```python
from build123d import *

# Parameters (mm, degrees)
SKETCH_1_R      = 2.15
EXTRUDE_1_DEPTH = 20
FILLET_1_R      = 10
FILLET_2_R      = 50
FILLET_3_R      = 1


with BuildPart() as part:
    # ｽｹｯﾁ1 → ﾎﾞｽ - 押し出し1 (new body)
    with BuildSketch(Plane(origin=(0, 0, 0), x_dir=(1, 0, 0), z_dir=(0, 1, 0))):
        with BuildLine():
            Line((-30, -24.445436483), (-19.445436483, -24.445436483))
            ThreePointArc((-19.445436483, -24.445436483), (-18.602258519, -24.373828809), (-17.78323176, -24.161056851))
            ThreePointArc((-17.78323176, -24.161056851), (0, -30), (17.78323176, -24.161056851))
            ThreePointArc((17.78323176, -24.161056851), (24.321347518, -18.338417254), (15.909902577, -15.909902577))
            Line((15.909902577, -15.909902577), (14.849242405, -14.849242405))
            ThreePointArc((14.849242405, -14.849242405), (0, -21), (-14.849242405, -14.849242405))
            Line((-14.849242405, -14.849242405), (-15.909902577, -15.909902577))
            ThreePointArc((-15.909902577, -15.909902577), (-17.532019321, -14.82603882), (-19.445436483, -14.445436483))
            Line((-19.445436483, -14.445436483), (-30, -14.445436483))
            Line((-30, -14.445436483), (-30, -24.445436483))
        make_face()
        with Locations(Location((-19.445436483, -19.445436483, 0), (0, 0, 270))):
            Circle(SKETCH_1_R, mode=Mode.SUBTRACT)
        with Locations(Location((19.445436483, -19.445436483, 0), (0, 0, 90))):
            Circle(SKETCH_1_R, mode=Mode.SUBTRACT)
    extrude(amount=EXTRUDE_1_DEPTH)

    # ﾌｨﾚｯﾄ1
    # the kernel refuses this fillet: 10 mm, written as the material it adds along each edge
    with BuildSketch(Plane(origin=(17.78323176, 0, 24.161056851), x_dir=(-0.8339213468601729, 0, 0.5518833094512962), z_dir=(0, 1, 0))) as fillet_1_piece_1:
        with BuildLine():
            CenterArc((3.490042654, 9.987563289), FILLET_1_R, 240.094065847, 27.048110546)
            ThreePointArc((-1.495732566, 1.319112133), (-0.681431037, 0.734886554), (0, 0))
            ThreePointArc((0, 0), (1.495732566, 0.037310133), (2.991465132, 0))
        make_face()
    extrude(amount=20)
    with BuildSketch(Plane(origin=(-17.78323176, 0, 24.161056851), x_dir=(-0.9938473156865714, 0, 0.11075880598217346), z_dir=(0, 1, 0))) as fillet_1_piece_2:
        with BuildLine():
            CenterArc((3.675145817, 9.938473157), FILLET_1_R, 233.085304015, 30.555636739)
            Line((-2.331107377, 1.943166873), (-2.931732696, 1.143636244))
            ThreePointArc((-2.931732696, 1.143636244), (-1.781263353, 0.232951381), (-0.678328899, -0.734758399))
            Line((-0.678328899, -0.734758399), (0.225936244, -0.974142091))
            ThreePointArc((0.225936244, -0.974142091), (1.572716444, -0.895321193), (2.456798951, -0.993847316))
            Line((2.456798951, -0.993847316), (2.567557757, 0))
        make_face()
    extrude(amount=20)
    # the kernel refuses this fillet: 10 mm, written as the material it takes off along each edge
    with BuildSketch(Plane(origin=(-14.849242405, -10.471736153, 14.849242405), x_dir=(-0.707106781186226, 0, 0.7071067811868691), z_dir=(0, 1, 0))) as fillet_1_2_piece_1:
        with BuildLine():
            CenterArc((9.383333333, 6.15248369), FILLET_1_R, 191.447340283, 26.522629156)
            ThreePointArc((-0.417741935, 4.167811532), (-0.104696468, 2.094347231), (0, 0))
            Line((0, 0), (1.5, 0))
        make_face()
    extrude(amount=40.943472307, mode=Mode.SUBTRACT)
    with BuildSketch(Plane(origin=(14.849242405, -10.471736153, 14.849242405), x_dir=(-0.7741018071953127, 0, 0.6330611282466734), z_dir=(0, 1, 0))) as fillet_1_2_piece_2:
        with BuildLine():
            CenterArc((5.186002666, 9.950144539), FILLET_1_R, 237.753700702, 26.522629156)
            Line((-0.149596231, 1.492521681), (0, 0))
            ThreePointArc((0, 0), (2.094347231, 0.104696468), (4.188694461, 0))
        make_face()
    extrude(amount=40.943472307, mode=Mode.SUBTRACT)

    # ﾌｨﾚｯﾄ2
    fillet_2_edges = [part.edges().sort_by_distance(p)[0] for p in [
        (-15.909902577, 10, 15.909902577),
        (15.909902577, 10, 15.909902577),
    ]]
    fillet(fillet_2_edges, radius=FILLET_2_R)

    # ﾌｨﾚｯﾄ3
    fillet_3_edges = [part.edges().sort_by_distance(p)[0] for p in [
        (-30, 10, 14.445436483),
        (-30, 10, 24.445436483),
    ]]
    fillet(fillet_3_edges, radius=FILLET_3_R)


solid = part.part
```
CAD build for the part. Positions are in the model's coordinates, mm. A direction names the side the tool comes from. Round coordinates to 2 decimals unless told otherwise and drop trailing zeros. Write each loop counter-clockwise with the first axis right and the second up, starting at its lowest first coordinate (ties: lowest second). Pieces come first, ordered by that corner, then holes. Notation, with made-up numbers: (38.25, 39.25) - (96.25, 39.25) arc R10 cw to (96.25, 58.25) - close; hole circle Ø10 at (6, -7.5). An arc over 180 degrees is marked (long way). Write item = value, one per line. Start each with the question number.
Q1. Band-saw the part on D-D (x = 6). Give the cut face in (y, z).
Q2. Band-saw the part on B-B (x = -18). Give the cut face in (y, z), then the cut area to 3 significant figures.
Q3. Probe L1, parallel to Z at x = 21, y = 17; L2, parallel to X at y = 14.25, z = 18; L3, parallel to Z at x = 20, y = 15. List the from-to ranges inside material, lowest first. Write a range as from..to.
Q4. Drop flat-ended pins along their axis: pin 1 (2.5 mm diameter, centred on x = -24.5, y = 13.5, fed in from +Z); pin 2 (8 mm diameter, centred on x = -2.5, y = 11, fed in from -Z); pin 3 (5 mm diameter, centred on x = -19.45, z = 19.45, fed in from -Y); pin 4 (2 mm diameter, centred on x = 14, y = 14.5, fed in from -Z). Give the stop position or say it passes through.
Q5. Band-saw the part on C-C (y = 12). Count the separate pieces of the cut face and the enclosed holes in it, then the cut area to 3 significant figures.
Q6. Mould opens along Z. For faces 4 (the cylindrical face through (0, 10, 21)), 5 (the cylindrical face through (17.63, 9.86, 18.29)), 6 (the flat face through (-30, 10, 19)) say: pulls with the +Z half, pulls with the -Z half, needs draft (parallel to the pull), parting line crosses it, or undercut.
Q7. Band-saw the part on A-A (z = 19.5). Give the cut face in (x, y), then the cut area to 3 significant figures.
Q8. Which spindle directions (+Z, -Z, +X, -X, +Y, -Y) get a long thin tool onto all of the face, cutting with end or side? Do faces 1 (the cylindrical face through (-18.345, 9.86, 14.568)), 2 (the cylindrical face through (-29.715, 10.14, 14.746)), 3 (the flat face through (-25, 10, 24.445)). Say none if no direction does.
Answers below:
q1.outline = (0, 20.12) - (20, 20.12) - (20, 29.39) - (0, 29.39) - close
q2.outline = (0, 14.66) - (20, 14.66) - (20, 17.85) - (0, 17.85) - close; (0, 21.04) - (20, 21.04) - (20, 24.72) - (0, 24.72) - close
q2.area = 138 mm2
q3.L1 = 14.69..17.96, 20.93..24.2
q3.L2 = -30..-21.04, -17.85..-10.82, 10.82..17.85, 21.04..24.23
q3.L3 = 14.48..17.37, 21.52..24.41
q4.pin_1 = 24.45
q4.pin_2 = 19.97
q4.pin_3 = 0
q4.pin_4 = 15.93
q5.separate_pieces = 1
q5.enclosed_holes = 2
q5.area = 491 mm2
q6.face_4 = pulls with the -Z half
q6.face_5 = undercut
q6.face_6 = needs draft
q7.outline = (-30, 0) - (-21.59, 0) - (-21.59, 20) - (-30, 20) - close; (-17.3, 0) - (-7.79, 0) - (-7.79, 20) - (-17.3, 20) - close; (7.79, 0) - (17.3, 0) - (17.3, 20) - (7.79, 20) - close; (21.59, 0) - (24.45, 0) - (24.45, 20) - (21.59, 20) - close
q7.area = 605 mm2
q8.face_1 = -Z, +Y, -Y
q8.face_2 = -Z, -X, +Y, -Y
q8.face_3 = +Z, -X, +Y, -Y
